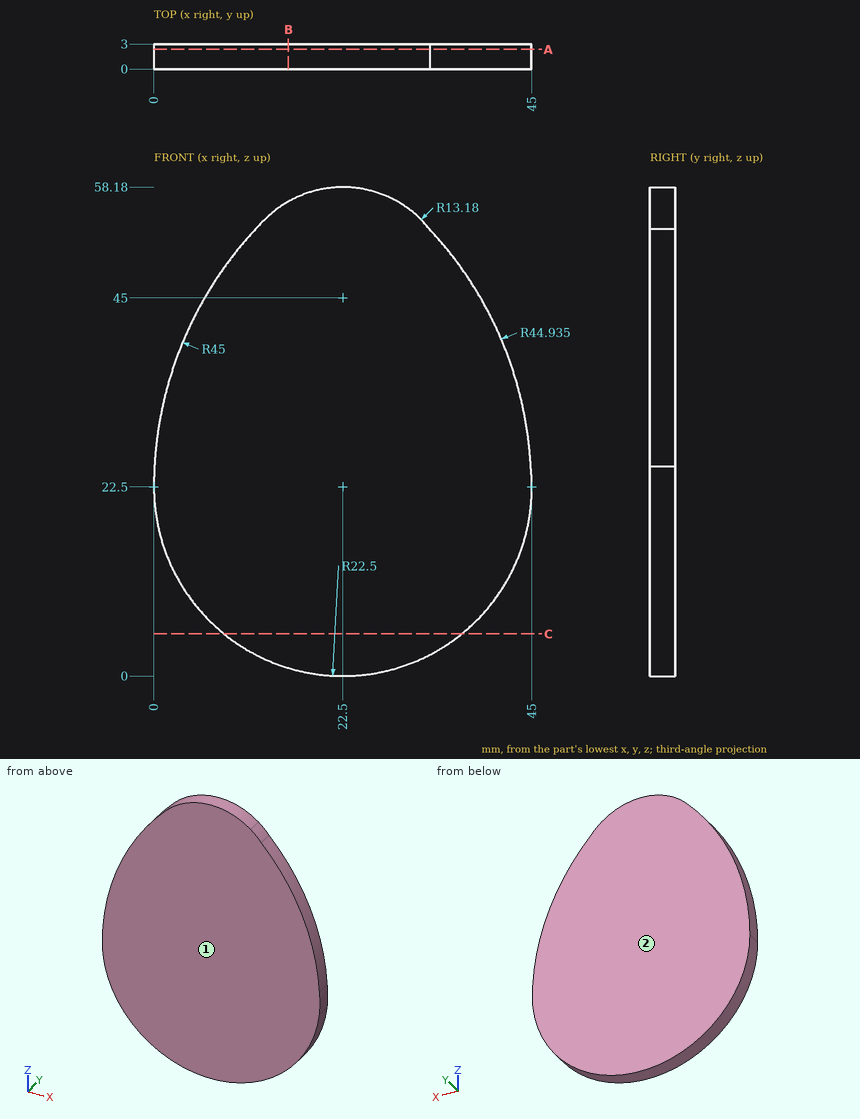
Source: three-view drawing plus pictorial views. Frame: mm from the lowest corner of the part. Give positions to 0.01 mm unless a question says otherwise; leave off trailing zeros. Write each loop counter-clockwise with the first axis right and the second up, starting at its lowest first coordinate (ties: lowest second). Pieces come first, ordered by that corner, then holes.
(1) Mould query, pull axis Y, two halves, no side actions, for the marked faces 1 and 2. Classes: released by +Y, released by -Y, zero draft, split by the parting line, or undercut.
(2) Cut plane C-C, the plane z = 5. Return loops of the section in (x, y).
(3) Ray query, line 1 (Z direction, x = 7.5, y = 2.3) (1 decimal); line 2 (Z direction, x = 34, y = 1.7); line 3 (X direction, y = 1.95, z = 25.5) (1 decimal). Return the intervals inside material, ascending.
(4) Cut plane B-B, the plane x = 16. Return loops of the section in (y, z).
(5) Cut plane A-A, the plane y = 2.35. Return loops of the section in (x, z) (1 decimal), then the cut area to 3 significant figures.
Values follow:
1. face 1: released by -Y
1. face 2: released by +Y
2. outline: (8.36, 0) - (36.64, 0) - (36.64, 3) - (8.36, 3) - close
3. line 1: z = 5.7 to 47.4
3. line 2: z = 3.16 to 51.88
3. line 3: x = 0.1 to 44.8
4. outline: (0, 0.96) - (3, 0.96) - (3, 56.47) - (0, 56.47) - close
5. outline: (0, 22.5) arc R22.5 ccw to (44.9, 20.1) arc R22.5 ccw to (44.9, 24.9) arc R44.9 ccw to (32.9, 53.2) arc R13.2 ccw to (30.7, 55.4) arc R13.2 ccw to (13.2, 54.3) arc R45 ccw to start
5. area: 2,010 mm2
